The figure shows three views and two pictorial views of one solid part (mm, origin at its lowest corner). Answer the questions. Round coordinates to 2 decimals unless told otherwise and drop trailing zeros. Order: outer loops, then holes, each group sorted by start corner. A loop starts at its lowest first (then second) coordinate and runs counter-clockwise, first axis right, second up. Notation, with made-up numbers: (2, -3) - (20, -3) arc R15 ccw to (20, 8) - close; hole circle Ø5 at (56, -6.75). An arc over 180 degrees is marked (long way). Write item = value, one per line.
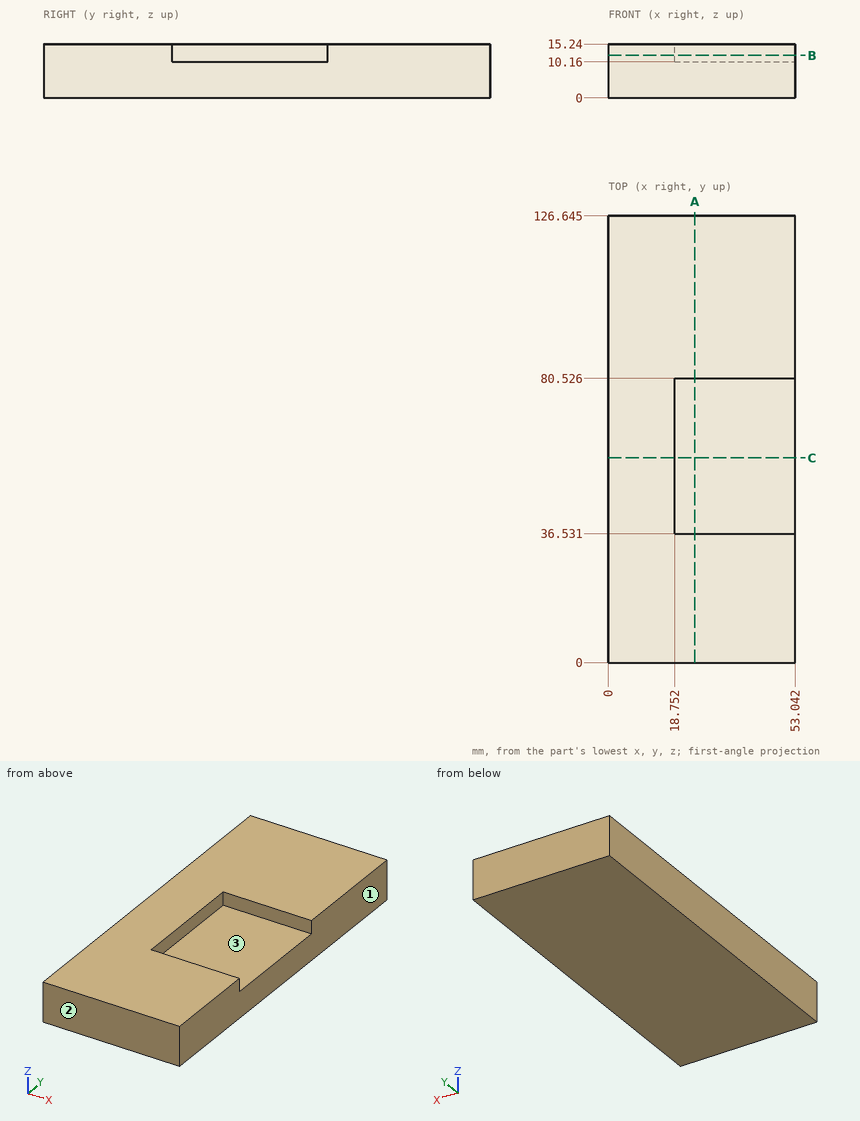
Q1. Find the intervals of material crossed by line 1 (Y direction, x = 39.5, z = 14) (1 decimal); line 2 (Z direction, x = 25, y = 40), in increasing order. Write a range as from..to.
Model answer:
line_1 = 0..36.5, 80.5..126.6
line_2 = 0..10.16
Q2. Determine the mould class of the marked faces 1, 2 and 3 for opening direction Y: released by +Y, released by -Y, zero draft, split by the parting line, or undercut.
Model answer:
face_1 = zero draft
face_2 = released by -Y
face_3 = undercut
Q3. Section A-A on x = 24.5 is taken. Determine the outline of the cut face in (y, z) (1 decimal).
Model answer:
outline = (0, 0) - (126.6, 0) - (126.6, 15.2) - (80.5, 15.2) - (80.5, 10.2) - (36.5, 10.2) - (36.5, 15.2) - (0, 15.2) - close
Q4. Section C-C on y = 58 is taken. Determine the outline of the cut face in (x, z), then the cut area to 3 significant figures.
Model answer:
outline = (0, 0) - (53.04, 0) - (53.04, 10.16) - (18.75, 10.16) - (18.75, 15.24) - (0, 15.24) - close
area = 634 mm^2
Q5. Section B-B on z = 12 is taken. Determine the outline of the cut face in (x, y) (1 decimal).
Model answer:
outline = (0, 0) - (53, 0) - (53, 36.5) - (18.8, 36.5) - (18.8, 80.5) - (53, 80.5) - (53, 126.6) - (0, 126.6) - close
Q6. Flat-ended cylindrical pins translate along their axes: P1, Ø17, axis at x = 32, y = 48, coming from the +Z side; P2, Ø2.5, axis at y = 61.5, z = 13, coming from the +X side. Find the tip coordinate at first contact, or state that the pin passes through.
Model answer:
P1 = 10.16
P2 = 18.75
